from build123d import *

# Parameters (mm, degrees)
SKETCH1_W            = 160.5788
SKETCH1_H            = 37.338
BOSS_EXTRUDE1_DEPTH  = 24.13
SKETCH2_W            = 157.5308
SKETCH2_H            = 34.29
CUT_EXTRUDE3_DEPTH   = 22.479
FILLET1_R            = 2.54
FILLET2_R            = 1.27
CUT_EXTRUDE4_REACH   = 165.451
SKETCH4_W            = 159.0548
SKETCH4_H            = 35.814
CUT_EXTRUDE5_DEPTH   = 1.778
FILLET3_R            = 1.524
SKETCH5_W            = 5.08
SKETCH5_H            = 0.762
BOSS_EXTRUDE2_DEPTH  = 7.62
SKETCH6_W            = 0.762
SKETCH6_H            = 2.032
BOSS_EXTRUDE3_DEPTH  = 25.019
LPATTERN1_COUNT      = 2
LPATTERN1_PITCH      = 101.6
LPATTERN1_COUNT_DIR2 = 2
LPATTERN1_PITCH_DIR2 = 32.258
CUT_EXTRUDE6_REACH   = 136.021
SKETCH8_W            = 3.81
SKETCH8_H            = 2.032
BOSS_EXTRUDE4_DEPTH  = 26.289
BOSS_EXTRUDE9_DEPTH  = 3.81
FILLET4_R            = 0.254
FILLET4_OF_MIRROR2_R = 0.254
SKETCH10_R           = 0.889
SKETCH10_W           = 23.114
SKETCH10_H           = 23.114
CUT_EXTRUDE7_DEPTH   = 88.711117296


with BuildPart() as part:
    # Sketch1 → Boss-Extrude1 (new body)
    with BuildSketch(Plane(origin=(0, 0, 0), x_dir=(1, 0, 0), z_dir=(0, 1, 0))):
        Rectangle(SKETCH1_W, SKETCH1_H)
    extrude(amount=BOSS_EXTRUDE1_DEPTH)

    # Sketch2 → Cut-Extrude3 (cut)
    with BuildSketch(Plane(origin=(0, 24.13, 0), x_dir=(1, 0, 0), z_dir=(0, 1, 0))):
        Rectangle(SKETCH2_W, SKETCH2_H)
    extrude(amount=-CUT_EXTRUDE3_DEPTH, mode=Mode.SUBTRACT)

    # Fillet1
    fillet1_edges = [part.edges().sort_by_distance(p)[0] for p in [
        (0, 0, 18.669),
        (-80.2894, 0, 0),
        (0, 0, -18.669),
        (80.2894, 0, 0),
        (80.2894, 12.065, 18.669),
        (-80.2894, 12.065, 18.669),
        (-80.2894, 12.065, -18.669),
        (80.2894, 12.065, -18.669),
    ]]
    fillet(fillet1_edges, radius=FILLET1_R)

    # Fillet2
    fillet2_edges = [part.edges().sort_by_distance(p)[0] for p in [
        (-78.7654, 12.8905, -17.145),
        (-78.7654, 12.8905, 17.145),
        (78.7654, 12.8905, 17.145),
        (78.7654, 12.8905, -17.145),
    ]]
    fillet(fillet2_edges, radius=FILLET2_R)

    # Sketch3 → Cut-Extrude4 (cut, up to next)
    with BuildSketch(Plane.ZY.offset(80.2894), mode=Mode.PRIVATE) as cut_extrude4_sk1:
        with BuildLine():
            Line((3.81, 15.2933146), (-3.81, 15.2933146))
            ThreePointArc((-3.81, 15.2933146), (-7.366, 18.8493146), (-3.81, 22.4053146))
            Line((-3.81, 22.4053146), (3.81, 22.4053146))
            ThreePointArc((3.81, 22.4053146), (7.366, 18.8493146), (3.81, 15.2933146))
        make_face()
    cut_extrude4_tool1 = extrude(cut_extrude4_sk1.sketch, amount=-CUT_EXTRUDE4_REACH, mode=Mode.PRIVATE) & part.part
    add(cut_extrude4_tool1.solids().sort_by_distance((-80.2894, 18.849315, 0))[0], mode=Mode.SUBTRACT)

    # Sketch4 → Cut-Extrude5 (cut)
    with BuildSketch(Plane(origin=(0, 24.13, 0), x_dir=(1, 0, 0), z_dir=(0, 1, 0))):
        Rectangle(SKETCH4_W, SKETCH4_H)
    extrude(amount=-CUT_EXTRUDE5_DEPTH, mode=Mode.SUBTRACT)

    # Fillet3
    fillet3_edges = [part.edges().sort_by_distance(p)[0] for p in [
        (-79.5274, 23.241, 17.907),
        (-79.5274, 23.241, -17.907),
        (79.5274, 23.241, -17.907),
        (79.5274, 23.241, 17.907),
    ]]
    fillet(fillet3_edges, radius=FILLET3_R)

    # Sketch5 → Boss-Extrude2 (add)
    with BuildSketch(Plane(origin=(0, 22.352, 0), x_dir=(1, 0, 0), z_dir=(0, 1, 0))):
        with Locations((-74.9554, -17.526)):
            Rectangle(SKETCH5_W, SKETCH5_H)
    extrude(amount=BOSS_EXTRUDE2_DEPTH)

    # Sketch6 → Boss-Extrude3 (add)
    with BuildSketch(Plane(origin=(0, 1.651, 0), x_dir=(1, 0, 0), z_dir=(0, 1, 0))):
        with Locations((-52.9844, 16.129)):
            Rectangle(SKETCH6_W, SKETCH6_H)
    boss_extrude3 = extrude(amount=BOSS_EXTRUDE3_DEPTH)

    # LPattern1: Boss-Extrude3 2 × 2
    with Locations(*[(i * LPATTERN1_PITCH, 0, j * LPATTERN1_PITCH_DIR2) for i in range(LPATTERN1_COUNT) for j in range(LPATTERN1_COUNT_DIR2) if (i, j) != (0, 0)]):
        add(boss_extrude3)

    # Cut-Extrude6: up to this face of the body (flat: up to its plane)
    cut_extrude6_end = Plane(part.part.faces().sort_by_distance((-53.3654, 14.1605, -16.129))[0])
    # Sketch7 → Cut-Extrude6 (cut, up to the picked face)
    with BuildSketch(Plane(origin=(48.9966, 0, 0), x_dir=(0, 0, -1), z_dir=(1, 0, 0)), mode=Mode.PRIVATE) as cut_extrude6_sk1:
        Polygon((17.145, 22.352), (15.494, 26.67), (17.145, 26.67), align=None)
    cut_extrude6_tool1 = split(extrude(cut_extrude6_sk1.sketch, amount=-CUT_EXTRUDE6_REACH, mode=Mode.PRIVATE), bisect_by=cut_extrude6_end, keep=Keep.BOTH, mode=Mode.PRIVATE)
    cut_extrude6 = cut_extrude6_tool1.solids().sort_by(Axis((48.9966, 25.230667, -16.594667), (-1, 0, 0)))[0]
    add(cut_extrude6, mode=Mode.SUBTRACT)

    # Mirror1: Cut-Extrude6 across plane
    add(cut_extrude6.mirror(Plane.XY), mode=Mode.SUBTRACT)

    # Sketch8 → Boss-Extrude4 (add)
    with BuildSketch(Plane(origin=(0, 1.651, 0), x_dir=(1, 0, 0), z_dir=(0, 1, 0))):
        with Locations((0, -16.129)):
            Rectangle(SKETCH8_W, SKETCH8_H)
        with Locations((0, 16.129)):
            Rectangle(SKETCH8_W, SKETCH8_H)
    extrude(amount=BOSS_EXTRUDE4_DEPTH)

    # Sketch9 → Boss-Extrude9 (add)
    with BuildSketch(Plane(origin=(1.905, 0, 0), x_dir=(0, 0, -1), z_dir=(1, 0, 0))):
        Polygon((-15.113, 27.94), (-17.907, 27.94), (-15.113, 29.972), align=None)
    boss_extrude9 = extrude(amount=-BOSS_EXTRUDE9_DEPTH)

    # Fillet4
    fillet4_edges = [part.edges().sort_by_distance(p)[0] for p in [
        (0, 29.972, 15.113),
    ]]
    fillet(fillet4_edges, radius=FILLET4_R)

    # Mirror2: Boss-Extrude9 across plane
    add(boss_extrude9.mirror(Plane.XY))

    # Fillet4 of Mirror2
    fillet4_of_mirror2_edges = [part.edges().sort_by_distance(p)[0] for p in [
        (0, 29.972, -15.113),
    ]]
    fillet(fillet4_of_mirror2_edges, radius=FILLET4_OF_MIRROR2_R)

    # Sketch10 → Cut-Extrude7 (cut, through all)
    with BuildSketch(Plane.XZ):
        with Locations(Location((-13.589, 0, 0), (0, 0, 270))):
            Circle(SKETCH10_R)
        with Locations(Location((13.589, 0, 0), (0, 0, 270))):
            Circle(SKETCH10_R)
        Rectangle(SKETCH10_W, SKETCH10_H)
    extrude(amount=-CUT_EXTRUDE7_DEPTH, mode=Mode.SUBTRACT)


solid = part.part
Check sheet for the modelled part. Datum: model origin and axes. Units: mm. A direction names the side the tool comes from. Coordinates: 2 decimals unless noted, no trailing zeros. Write each loop counter-clockwise with the first axis right and the second up, starting at its lowest first coordinate (ties: lowest second). Pieces come first, ordered by that corner, then holes.
Item 1: Cross-section at A-A on x = 6.5. Record the boundary of the cut face in (y, z) (3 decimals).
Numbers:
outline: (0, -16.129) arc R2.54 ccw to (2.54, -18.669) - (24.13, -18.669) - (24.13, -17.907) - (22.352, -17.907) - (22.352, -17.145) - (1.651, -17.145) - (1.651, -11.557) - (0, -11.557) - close; (0, 11.557) - (1.651, 11.557) - (1.651, 17.145) - (22.352, 17.145) - (22.352, 17.907) - (24.13, 17.907) - (24.13, 18.669) - (2.54, 18.669) arc R2.54 ccw to (0, 16.129) - close
Item 2: Mould release check, pull along Z, two halves, no side actions. Record for faces 6 (the face through (-79.6, 0.8, -0.2)), 7 (the face through (0, 25, -17.145)), 8 (the face through (-79.565, 13.486, -17.905)), 9 (the face through (1.09, 0.76, 17.94)): released by +Z, released by -Z, zero draft, split by the parting line, or undercut.
Numbers:
face 6: zero draft
face 7: undercut
face 8: released by -Z
face 9: released by +Z
Item 3: Cross-section at B-B on x = 56. Record the boundary of the cut face in (y, z) (3 decimals).
Numbers:
outline: (0, -16.129) arc R2.54 ccw to (2.54, -18.669) - (24.13, -18.669) - (24.13, -17.907) - (22.352, -17.907) - (22.352, -17.145) - (1.651, -17.145) - (1.651, 17.145) - (22.352, 17.145) - (22.352, 17.907) - (24.13, 17.907) - (24.13, 18.669) - (2.54, 18.669) arc R2.54 ccw to (0, 16.129) - close
Item 4: Access from +Z, -Z, +X, -X, +Y, -Y to the whole of each face (thin tool, end or side, straight path). Record for faces 1 (the face through (-79.538, 18.928, 7.365)), 2 (the face through (0, 25, 17.145)), 3 (the face through (80.289, 13, 0)), 4 (the face through (79.5, 0.7, -0.2)), 5 (the face through (25, 12, -17.145)).
Numbers:
face 1: -X
face 2: none
face 3: +Z, -Z, +X, +Y, -Y
face 4: +Z, -Z, +X, -Y
face 5: +Y
Item 5: Depth check by flat-ended pin: pin 1 Ø8 at (x, z) = (35.5, -6.5) entering from +Y; pin 2 Ø1.6 at (x, z) = (-78, 14) entering from +Y; pin 3 Ø1.1 at (x, y) = (1, 25) entering from -Z (3 decimals). Enter the tip coordinate at first touch or a pass-through.
Numbers:
pin 1: stops at y = 1.65
pin 2: stops at y = 22.35
pin 3: stops at z = -17.145
Item 6: Scan lines: probe 1 along X at (y, z) = (0.7, 0); probe 2 along X at (y, z) = (5, -11.5); probe 3 along Z at (x, y) = (29, 21.25) (3 decimals). Record each from-to range of solid material in increasing order.
Numbers:
probe 1: x = -79.5 to -14.48, -12.7 to -11.56, 11.56 to 12.7, 14.48 to 79.5
probe 2: x = -80.29 to -78.77, 78.77 to 80.29
probe 3: z = -18.669 to -17.145, 17.145 to 18.669
